The listing builds one solid part. Answer for the finished solid, in the listing's coordinates (mm). Face numbers are marked on the shaded views. A direction names the side the tool comes from. Give positions to 0.01 mm unless a question says otherwise; leave off trailing zeros. Write each loop counter-clockwise with the first axis right and the second up, starting at its lowest first coordinate (ties: lowest second). Pieces come first, ordered by that corner, then holes. Notation, with made-up numbers: (-24.5, 51.5) - (-6.5, 51.5) arc R25 cw to (-6.5, 90.5) - close; hole circle Ø3 at (75.5, 29.5). An arc over 180 degrees is marked (long way). Write each question's results on one line, items separated by ' | '. Start each with the question number.
Q1. Find the intervals of material crossed by probe 1 along X at (y, z) = (-15, 16); probe 2 along X at (y, z) = (-15, -1); probe 3 along Y at (x, z) = (5.75, 32), in increasing order.
Q2. For a pull along Z with two mould halves and no side action, classify the marked faces 6, 7 and 8 as pulls with the +Z half, pulls with the -Z half, needs draft (parallel to the pull), parting line crosses it, or undercut.
Q3. Section A-A (y = -15) is taken. Determine the outline of the cut face in (x, z).
Q4. For the marked faces 1, 2, 3, 4 and 5, determine the directions among +Z, -Z, +X, -X, +Y, -Y from which every point of the face is accessible in a straight line to the end or side of a thin tool.
Q5. Section B-B (z = 20.5) is taken. Determine the outline of the cut face in (x, y).
Q6. Section D-D (x = 48.5) is taken. Determine the outline of the cut face in (y, z).
Q7. Section C-C (x = 30) is taken. Determine the outline of the cut face in (y, z), plus the area to 3 significant figures.
Q8. Flat-ended cylindrical pins translate along their axes: pin 1 Ø6 at (x, y) = (41.5, -23) entering from +Z; pin 2 Ø6.5 at (x, z) = (10.5, 21.5) entering from +Y; pin 3 Ø1 at (x, z) = (29, 6) entering from +Y. Find the tip coordinate at first contact, or state that the pin passes through.
```python
from build123d import *

# Parameters (mm, degrees)
F1_DEPTH      = 30
F2_R          = 17
F3_DEPTH      = 10
F3_DEPTH_BACK = 6
F4_R          = 10
F5_DEPTH      = 25
F5_DEPTH_BACK = 25
F6_R          = 7.5
F7_DEPTH      = 70


with BuildPart() as f1:
    # F0 (on Front) → F1 (new body)
    with BuildSketch(Plane.XZ):
        Polygon((0, 47), (0, 0), (55, 0), (55, 47), (45, 47), (45, 10), (10, 10), (10, 47), align=None)
    extrude(amount=F1_DEPTH)

    # F2 (on Top) → F3 (join, two sides)
    with BuildSketch(Plane.XY) as f3_sk:
        with Locations((30, -15)):
            Circle(F2_R)
    extrude(amount=F3_DEPTH)
    extrude(f3_sk.sketch, amount=-F3_DEPTH_BACK)

    # F4 (on Top) → F5 (cut, two sides)
    with BuildSketch(Plane.XY) as f5_sk:
        with Locations((30, -15)):
            Circle(F4_R)
    extrude(amount=-F5_DEPTH, mode=Mode.SUBTRACT)
    extrude(f5_sk.sketch, amount=F5_DEPTH_BACK, mode=Mode.SUBTRACT)

    # F6 (on Right) → F7 (cut)
    with BuildSketch(Plane.YZ):
        with BuildLine():
            ThreePointArc((-30, 32), (-25.6066017178, 42.6066017178), (-15, 47))
            Line((-15, 47), (-30, 47))
            Line((-30, 47), (-30, 32))
        make_face()
        with BuildLine():
            ThreePointArc((-15, 47), (-4.3933982822, 42.6066017178), (0, 32))
            Line((0, 32), (0, 47))
            Line((0, 47), (-15, 47))
        make_face()
        with Locations((-15, 32)):
            Circle(F6_R)
    extrude(amount=F7_DEPTH, mode=Mode.SUBTRACT)


solid = f1.part
```
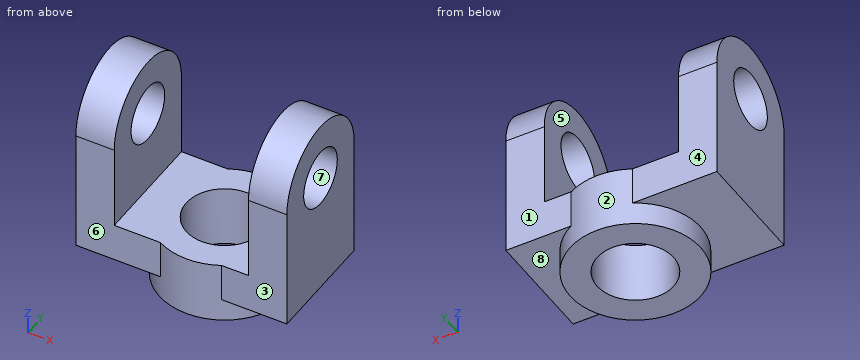
Answers below:
1) probe 1: x = 0 to 10, 45 to 55 | probe 2: x = 13 to 20, 40 to 47 | probe 3: y = -30 to -22.5, -7.5 to 0
2) face 6: needs draft | face 7: undercut | face 8: pulls with the -Z half
3) outline: (0, 0) - (13, 0) - (13, -6) - (20, -6) - (20, 10) - (10, 10) - (10, 24.5) - (0, 24.5) - close; (0, 39.5) - (10, 39.5) - (10, 47) - (0, 47) - close; (40, -6) - (47, -6) - (47, 0) - (55, 0) - (55, 24.5) - (45, 24.5) - (45, 10) - (40, 10) - close; (45, 39.5) - (55, 39.5) - (55, 47) - (45, 47) - close
4) face 1: +Z, -Z, +X, +Y | face 2: -Z | face 3: +Z, -Z, +X, -Y | face 4: +Z, -Z, -X, +Y | face 5: +Z, +Y, -Y
5) outline: (0, -30) - (10, -30) - (10, 0) - (0, 0) - close; (45, -30) - (55, -30) - (55, 0) - (45, 0) - close
6) outline: (-30, 0) - (0, 0) - (0, 32) arc R15 ccw to (-30, 32) - close; hole circle Ø15 at (-15, 32)
7) outline: (-32, -6) - (-25, -6) - (-25, 10) - (-32, 10) - close; (-5, -6) - (2, -6) - (2, 10) - (-5, 10) - close | area: 224 mm2
8) pin 1: stops at z = 10 | pin 2: stops at y = 0 | pin 3: stops at y = 1.99
